The model under review builds one solid part; all positions refer to its coordinate system, in mm. Coordinates: 2 decimals unless noted, no trailing zeros. Order: outer loops, then holes, each group sorted by start corner. A loop starts at its lowest first (then second) coordinate and runs counter-clockwise, first axis right, second up. Notation, with made-up numbers: M 71,0 L 90,0 A28 cw 90,21 Z; hole C 35.25,25 d8. An arc over 180 degrees is marked long. One line per item, written item: value.
```python
from build123d import *

# Parameters (mm, degrees)
SKETCH1_W           = 275
SKETCH1_H           = 175
BOSS_EXTRUDE1_DEPTH = 25
FILLET1_R           = 10
SKETCH2_R           = 5
CUT_EXTRUDE1_DEPTH  = 180
CUT_EXTRUDE2_DEPTH  = 125
SKETCH5_R           = 5
CUT_EXTRUDE3_DEPTH  = 190
BOSS_EXTRUDE2_START = 30
SKETCH6_R           = 7
SKETCH6_R_2         = 5
BOSS_EXTRUDE2_DEPTH = 30
BOSS_EXTRUDE3_START = 30
SKETCH7_R           = 7
SKETCH7_R_2         = 5
BOSS_EXTRUDE3_DEPTH = 30


with BuildPart() as part:
    # Sketch1 → Boss-Extrude1 (new, symmetric)
    with BuildSketch(Plane.XY):
        Rectangle(SKETCH1_W, SKETCH1_H)
    extrude(amount=BOSS_EXTRUDE1_DEPTH, both=True)

    # Fillet1
    fillet1_edges = [part.edges().sort_by_distance(p)[0] for p in [
        (137.5, 0, 25),
        (0, 87.5, 25),
        (-137.5, 0, 25),
        (0, 87.5, -25),
        (137.5, 0, -25),
        (0, -87.5, -25),
        (-137.5, 0, -25),
        (-137.5, 87.5, 0),
        (137.5, 87.5, 0),
        (137.5, -87.5, 0),
        (-137.5, -87.5, 0),
        (0, -87.5, 25),
    ]]
    fillet(fillet1_edges, radius=FILLET1_R)

    # Sketch2 → Cut-Extrude1 (cut)
    with BuildSketch(Plane(origin=(137.5, 0, 0), x_dir=(0, 0, -1), z_dir=(1, 0, 0))):
        with Locations((0, 75)):
            Circle(SKETCH2_R)
        with Locations((0, 25)):
            Circle(SKETCH2_R)
        with Locations((0, -75)):
            Circle(SKETCH2_R)
    extrude(amount=-CUT_EXTRUDE1_DEPTH, mode=Mode.SUBTRACT)

    # Sketch3 → Cut-Extrude2 (cut, symmetric)
    with BuildSketch(Plane(origin=(0, 0, 0), x_dir=(0, 0, -1), z_dir=(1, 0, 0))):
        with BuildLine():
            Line((-15, 82.5), (15, 82.5))
            ThreePointArc((15, 82.5), (18.535533906, 81.035533906), (20, 77.5))
            Line((20, 77.5), (20, -77.567792301))
            ThreePointArc((20, -77.567792301), (18.535533906, -81.103326207), (15, -82.567792301))
            Line((15, -82.567792301), (-15, -82.567792301))
            ThreePointArc((-15, -82.567792301), (-18.535533906, -81.103326207), (-20, -77.567792301))
            Line((-20, -77.567792301), (-20, 77.5))
            ThreePointArc((-20, 77.5), (-18.535533906, 81.035533906), (-15, 82.5))
        make_face()
    extrude(amount=CUT_EXTRUDE2_DEPTH, both=True, mode=Mode.SUBTRACT)

    # Sketch5 → Cut-Extrude3 (cut)
    with BuildSketch(Plane.ZY.offset(137.5)):
        with Locations((0, -50)):
            Circle(SKETCH5_R)
    extrude(amount=-CUT_EXTRUDE3_DEPTH, mode=Mode.SUBTRACT)

    # Sketch6 → Boss-Extrude2 (add)
    with BuildSketch(Plane(origin=(137.5, 0, 0), x_dir=(0, 0, -1), z_dir=(1, 0, 0)).offset(BOSS_EXTRUDE2_START)):
        with Locations(Location((0, 25, 0), (0, 0, 180))):
            Circle(SKETCH6_R)
        with Locations((0, 25)):
            Circle(SKETCH6_R_2, mode=Mode.SUBTRACT)
    extrude(amount=-BOSS_EXTRUDE2_DEPTH)

    # Sketch7 → Boss-Extrude3 (add)
    with BuildSketch(Plane.ZY.offset(137.5).offset(BOSS_EXTRUDE3_START)):
        with Locations(Location((0, -50, 0), (0, 0, 180))):
            Circle(SKETCH7_R)
        with Locations((0, -50)):
            Circle(SKETCH7_R_2, mode=Mode.SUBTRACT)
    extrude(amount=-BOSS_EXTRUDE3_DEPTH)


solid = part.part
```
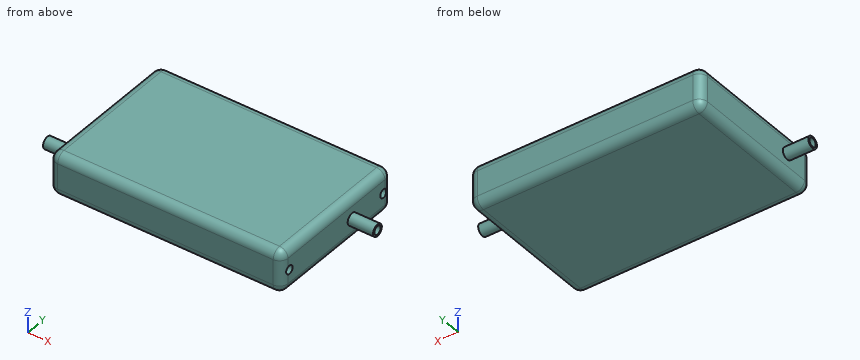
(1) We need section D-D, the plane z = 0. Count the separate pieces of the cut face and the enclosed holes in it, plus the area to 3 significant figures.
Geometry results:
separate pieces: 4
enclosed holes: 0
area: 6,510 mm2
(2) We need section A-A, the plane y = 55.5. State the section outline as (x, z) points.
Geometry results:
outline: M -137.5,-15 A10 ccw -127.5,-25 L 127.5,-25 A10 ccw 137.5,-15 L 137.5,15 A10 ccw 127.5,25 L -127.5,25 A10 ccw -137.5,15 Z; hole M -125,-20 L 125,-20 L 125,20 L -125,20 Z
(3) We need section C-C, the plane y = -50. State the section outline as (x, z) points, plus the area to 3 significant figures.
Geometry results:
outline: M -167.5,-7 L -137.5,-7 L -137.5,-15 A10 ccw -127.5,-25 L 127.5,-25 A10 ccw 137.5,-15 L 137.5,15 A10 ccw 127.5,25 L -127.5,25 A10 ccw -137.5,15 L -137.5,7 L -167.5,7 L -167.5,5 L -125,5 L -125,20 L 125,20 L 125,-20 L -125,-20 L -125,-5 L -167.5,-5 Z
area: 3,660 mm2
(4) Insertion check: pin 1 Ø20 at (y, z) = (-19.5, 9) entering from +X; pin 2 Ø6 at (y, z) = (42.5, -16.5) entering from -X; pin 3 Ø9 at (y, z) = (-75, 0) entering from +X. Each pin has a flat end and moves straight along its axis. Give the tip position at first contact, or say it passes through.
Geometry results:
pin 1: stops at x = 137.5
pin 2: stops at x = -137.5
pin 3: stops at x = -125
(5) For L1, parallel to Y at x = 128.5, z = 0; L2, parallel to Y at x = -58.5, z = 6; L3, parallel to Z at x = 9, y = -58, list the stretches that pass through material, from the lowest coordinate up.
Geometry results:
L1: y = -87.45 to -80, -70 to 20, 30 to 70, 80 to 87.45
L2: y = -87.5 to -82.57, 82.5 to 87.5
L3: z = -25 to -20, 20 to 25
(6) We need section B-B, the plane x = -89.5. State the section outline as (y, z) points.
Geometry results:
outline: M -87.5,-15 A10 ccw -77.5,-25 L 77.5,-25 A10 ccw 87.5,-15 L 87.5,15 A10 ccw 77.5,25 L -77.5,25 A10 ccw -87.5,15 Z; hole M -82.57,-15 A5 ccw -77.57,-20 L 77.5,-20 A5 ccw 82.5,-15 L 82.5,15 A5 ccw 77.5,20 L -77.57,20 A5 ccw -82.57,15 Z
